```python
from build123d import *

# Parameters (mm, degrees)
SKETCH1_R           = 18
SKETCH1_W           = 10
SKETCH1_H           = 3
SKETCH1_W_2         = 30
BOSS_EXTRUDE1_DEPTH = 3


with BuildPart() as part:
    # Sketch1 → Boss-Extrude1 (new body)
    with BuildSketch(Plane.XY):
        with BuildLine():
            Line((-45, 10), (-45, -10))
            Line((-45, -10), (-48, -10))
            Line((-48, -10), (-48, -20))
            Line((-48, -20), (-45, -20))
            Line((-45, -20), (-45, -25))
            Line((-45, -25), (70, -25))
            Line((70, -25), (70, -15))
            ThreePointArc((70, -15), (67.071067812, -7.928932188), (60, -5))
            Line((60, -5), (45, -5))
            Line((45, -5), (45, 10))
            Line((45, 10), (48, 10))
            Line((48, 10), (48, 20))
            Line((48, 20), (45, 20))
            Line((45, 20), (45, 25))
            Line((45, 25), (-45, 25))
            Line((-45, 25), (-45, 20))
            Line((-45, 20), (-48, 20))
            Line((-48, 20), (-48, 10))
            Line((-48, 10), (-45, 10))
        make_face()
        Circle(SKETCH1_R, mode=Mode.SUBTRACT)
        with Locations((-30, 11.5)):
            Rectangle(SKETCH1_W, SKETCH1_H, mode=Mode.SUBTRACT)
        with Locations((50, -21.5)):
            Rectangle(SKETCH1_W_2, SKETCH1_H, mode=Mode.SUBTRACT)
    extrude(amount=BOSS_EXTRUDE1_DEPTH)


solid = part.part
```
Part model, mm, in its own coordinate system. A direction names the side the tool comes from. Give positions to 0.01 mm unless a question says otherwise; leave off trailing zeros. Write each loop counter-clockwise with the first axis right and the second up, starting at its lowest first coordinate (ties: lowest second). Pieces come first, ordered by that corner, then holes. Notation, with made-up numbers: M 76,-7 L 133,-7 A26 cw 133,17 Z; hole C 29.5,-15 d2. An arc over 180 degrees is marked long. Use CSV: the item, a comma, the result in double quotes.
Item 1: Slice it at A-A on x = 0. Write the cut outline in (y, z), plus the area to 3 significant figures.
Taken from the geometry:
outline,"M -25,0 L -18,0 L -18,3 L -25,3 Z; M 18,0 L 25,0 L 25,3 L 18,3 Z"
area,"42.0 mm²"
Item 2: Pull direction Y, two halves, no side cores. Call faces 1 (the face through (50, -20, 1)), 2 (the face through (46, 10, 1)), 3 (the face through (10, -16, 0)), 4 (the face through (-47, -20, 1)): +Y half, -Y half, draft (parallel to the pull), parting line (faces both ways), or undercut.
Taken from the geometry:
face 1,"undercut"
face 2,"undercut"
face 3,"draft"
face 4,"-Y half"
Item 3: Pin check, flat tips, straight feed: P1, Ø1, axis at y = 0.5, z = 1, coming from the +X side; P2, Ø1.5, axis at x = -46.5, z = 1.5, coming from the -Y side; P3, Ø0.9, axis at x = -46, z = 1.5, coming from the +Y side. Stop position of each tip, or through.
Taken from the geometry:
P1,"stops at x = 45"
P2,"stops at y = -20"
P3,"stops at y = 20"
Item 4: Drill centre lines: probe 1 along Y at (x, z) = (42, 2.65); probe 2 along Y at (x, z) = (-27, 2.35); probe 3 along X at (y, z) = (-21, 2.1). Where is each one in solid material? Low to high.
Taken from the geometry:
probe 1,"y = -25 to -23, -20 to 25"
probe 2,"y = -25 to 10, 13 to 25"
probe 3,"x = -45 to 35, 65 to 70"
Item 5: Slice it at C-C on z = 0.75. Write the cut outline in (x, y).
Taken from the geometry:
outline,"M -48,-20 L -45,-20 L -45,-25 L 70,-25 L 70,-15 A10 ccw 60,-5 L 45,-5 L 45,10 L 48,10 L 48,20 L 45,20 L 45,25 L -45,25 L -45,20 L -48,20 L -48,10 L -45,10 L -45,-10 L -48,-10 Z; hole M -35,10 L -25,10 L -25,13 L -35,13 Z; hole C 0,0 d36; hole M 35,-23 L 65,-23 L 65,-20 L 35,-20 Z"
Item 6: Slice it at B-B on y = 0. Write the cut outline in (x, z).
Taken from the geometry:
outline,"M -45,0 L -18,0 L -18,3 L -45,3 Z; M 18,0 L 45,0 L 45,3 L 18,3 Z"
Item 7: Which spindle directions (+Z, -Z, +X, -X, +Y, -Y) get a long thin tool onto all of the face, cutting with end or side? Do faces 5 (the face through (48, 15, 1)), 6 (the face through (-46, -10, 1)), 7 (the face through (-25, 11, 1)), 8 (the face through (53, -5, 1)). Say none if no direction does.
Taken from the geometry:
face 5,"+Z, -Z, +X, +Y"
face 6,"+Z, -Z, -X"
face 7,"+Z, -Z"
face 8,"+Z, -Z, +X"
